Verification items for this drawing (mm, ordinates from the low corner). A direction names the side the tool comes from. Round coordinates to 2 decimals unless told otherwise and drop trailing zeros. Write each loop counter-clockwise with the first axis right and the second up, starting at its lowest first coordinate (ties: lowest second). Pieces come first, ordered by that corner, then holes. Notation, with made-up numbers: (-40, -35) -> (-25, -35) arc R33 ccw to (-25, -1) -> close; hole circle Ø6 at (15.5, 49). An arc over 180 degrees is marked (long way). Put each result on its own line as item: value. Start each with the question number.
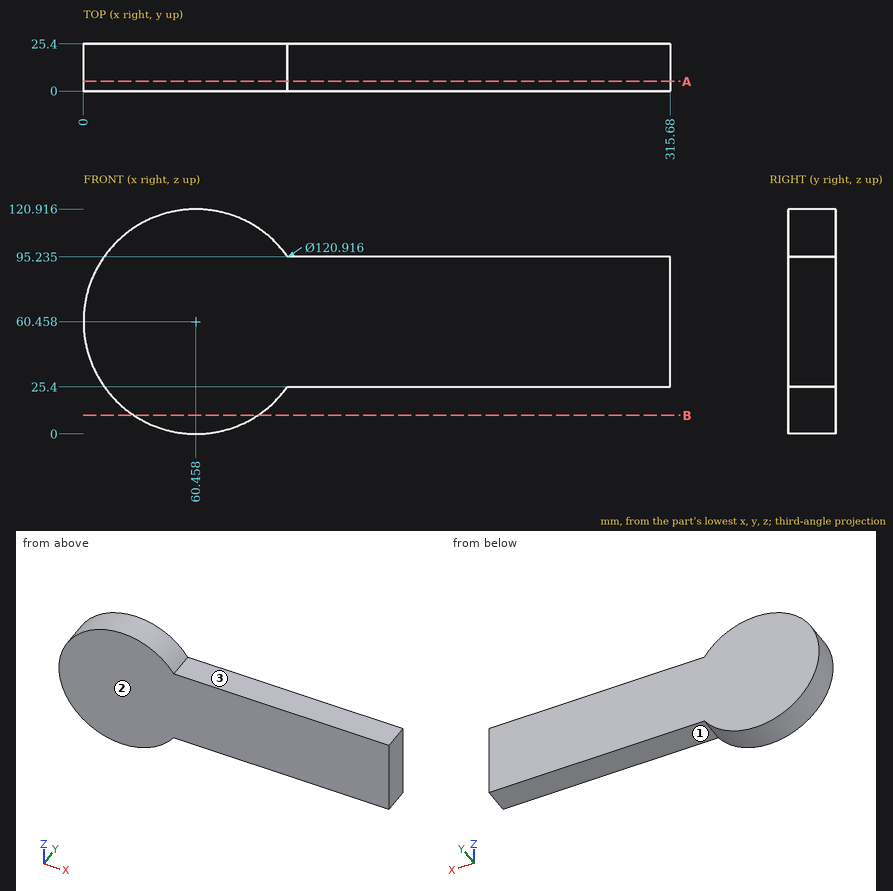
(1) Set-up check for the marked faces 1, 2 and 3: record each of +Z, -Z, +X, -X, +Y, -Y from which the full face is reachable in a straight line by a thin tool's end or side.
(2) Go/stop test with flat-tipped pins: pin 1 Ø7.5 at (x, y) = (180, 15) entering from -Z; pin 2 Ø12.5 at (x, y) = (254, 17.5) entering from +Z (1 decimal); pin 3 Ø12 at (x, y) = (93.5, 11.5) entering from -Z (1 decimal); pin 4 Ø1.5 at (x, z) = (42, 52) entering from -Y. Record where each tip stops, or that it passes through.
(3) Sectioned sample at A-A (y = 5.25). Record the cut outline in (x, z) (1 decimal).
(4) Material ranges on L1, parallel to Z at x = 176.5, y = 4.5 (1 decimal); L2, parallel to X at y = 1.5, z = 58.5; L3, parallel to X at y = 18.75, z = 63, recorded low to high. Write a range as from..to.
(5) Sectioned sample at B-B (z = 10). Record the cut outline in (x, y), and give its area (3 significant figures).
Found:
1. face 1: -Z, +X, +Y, -Y
1. face 2: +Z, -Z, +X, -X, -Y
1. face 3: +Z, +X, +Y, -Y
2. pin 1: z = 25.4
2. pin 2: z = 95.2
2. pin 3: z = 6.4
2. pin 4: y = 0
3. outline: (109.7, 25.4) -> (315.7, 25.4) -> (315.7, 95.2) -> (109.9, 95.2) arc R60.5 ccw (long way) to start
4. L1: 25.4..95.2
4. L2: 0.03..315.68
4. L3: 0.05..315.68
5. outline: (27.15, 0) -> (93.76, 0) -> (93.76, 25.4) -> (27.15, 25.4) -> close
5. area: 1,690 mm2
